Geometry check sheet. Reference: the model listing, model coordinates, mm. Face numbers are marked on the shaded views. Round coordinates to 2 decimals unless told otherwise and drop trailing zeros. Loops run counter-clockwise (first coordinate to the right, second up) from the corner with the lowest first, then second, coordinate; pieces in that order, holes last. Notation, with made-up numbers: (-13.5, -38.5) -> (18.5, -38.5) arc R21 ccw to (18.5, -21.5) -> close; hole circle Ø11 at (78.5, 38.5). An arc over 180 degrees is marked (long way). Use a Markdown table: item, result. Add a question column.
Q1. Sectioned sample at B-B, the plane x = -0.5. Give the number of separate pieces and of enclosed holes in the cut face, then the cut area to 3 significant figures.
Q2. Material ranges on L1, parallel to Z at x = -0.5, y = 1.9; L2, parallel to X at y = 1.95, z = 17.5; L3, parallel to Z at x = -0.5, y = 4.5, recorded low to high.
Q3. Sectioned sample at D-D, the plane z = 29. Enter the section's corners in (x, y), then the cut area to 3 significant figures.
Q4. Sectioned sample at C-C, the plane y = 6.25. Enter the section's corners in (x, z), then the cut area to 3 significant figures.
Q5. Gauge pin test, flat ends, axial feed: P1, Ø1, axis at y = 5, z = -16, coming from the +X side; P2, Ø5, axis at x = -1, z = -17.5, coming from the +Y side. Record the tip position at first contact, or that the pin passes through.
Q6. Release check for a two-part mould opening along Z. For the marked faces 1, 2, 3 and 4 record: released by +Z, released by -Z, zero draft, split by the parting line, or undercut.
Q7. Sectioned sample at A-A, the plane z = -6.5. Enter the section's corners in (x, y).
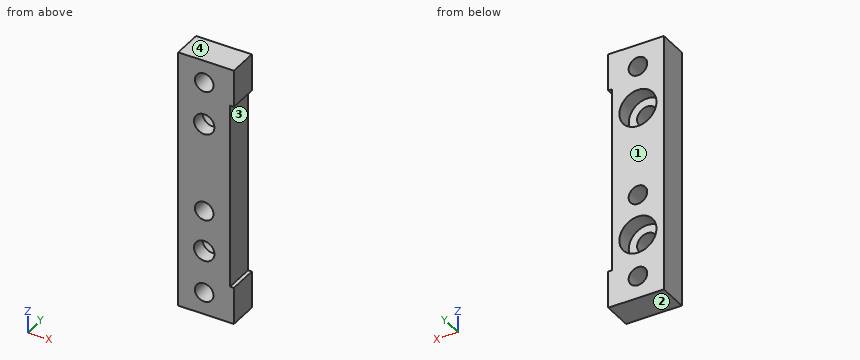
```python
from build123d import *

# Parameters (mm, degrees)
SKETCH1_W           = 15
SKETCH1_H           = 70
BOSS_EXTRUDE1_DEPTH = 8
SKETCH2_W           = 1
SKETCH2_H           = 50
CUT_EXTRUDE1_DEPTH  = 8
SKETCH3_R           = 2.5
CUT_EXTRUDE2_DEPTH  = 8
SKETCH4_R           = 2.75
CUT_EXTRUDE3_DEPTH  = 8
SKETCH5_R           = 5
CUT_EXTRUDE4_DEPTH  = 4.2
SKETCH6_R           = 2.5
CUT_EXTRUDE5_DEPTH  = 72.2


with BuildPart() as part:
    # Sketch1 → Boss-Extrude1 (new body)
    with BuildSketch(Plane(origin=(0, 0, 0), x_dir=(1, 0, 0), z_dir=(0, 1, 0))):
        Rectangle(SKETCH1_W, SKETCH1_H)
    extrude(amount=BOSS_EXTRUDE1_DEPTH)

    # Sketch2 → Cut-Extrude1 (cut)
    with BuildSketch(Plane(origin=(0, 8, 0), x_dir=(1, 0, 0), z_dir=(0, 1, 0))):
        with Locations((7, 0)):
            Rectangle(SKETCH2_W, SKETCH2_H)
    extrude(amount=-CUT_EXTRUDE1_DEPTH, mode=Mode.SUBTRACT)

    # Sketch3 → Cut-Extrude2 (cut)
    with BuildSketch(Plane(origin=(0, 8, 0), x_dir=(1, 0, 0), z_dir=(0, 1, 0))):
        with Locations((-0.5, -29)):
            Circle(SKETCH3_R)
        with Locations((-0.5, 29)):
            Circle(SKETCH3_R)
    extrude(amount=-CUT_EXTRUDE2_DEPTH, mode=Mode.SUBTRACT)

    # Sketch4 → Cut-Extrude3 (cut)
    with BuildSketch(Plane(origin=(0, 8, 0), x_dir=(1, 0, 0), z_dir=(0, 1, 0))):
        with Locations((-0.5, -17.5)):
            Circle(SKETCH4_R)
        with Locations((-0.5, 17.5)):
            Circle(SKETCH4_R)
    extrude(amount=-CUT_EXTRUDE3_DEPTH, mode=Mode.SUBTRACT)

    # Sketch5 → Cut-Extrude4 (cut)
    with BuildSketch(Plane(origin=(0, 8, 0), x_dir=(1, 0, 0), z_dir=(0, 1, 0))):
        with Locations((-0.5, 17.5)):
            Circle(SKETCH5_R)
        with Locations((-0.5, -17.5)):
            Circle(SKETCH5_R)
    extrude(amount=-CUT_EXTRUDE4_DEPTH, mode=Mode.SUBTRACT)

    # Sketch6 → Cut-Extrude5 (cut)
    with BuildSketch(Plane(origin=(0, 8, 0), x_dir=(1, 0, 0), z_dir=(0, 1, 0))):
        with Locations((-0.5, 6.5)):
            Circle(SKETCH6_R)
    extrude(amount=-CUT_EXTRUDE5_DEPTH, mode=Mode.SUBTRACT)


solid = part.part
```
Values:
| question | item | result |
|---|---|---|
| 1 | separate pieces | 6 |
| 1 | enclosed holes | 0 |
| 1 | area | 314 mm^2 |
| 2 | L1 | -35 to -31.5, -26.5 to -20.25, -14.75 to -9, -4 to 14.75, 20.25 to 26.5, 31.5 to 35 |
| 2 | L2 | -7.5 to -3.25, 2.25 to 6.5 |
| 2 | L3 | -35 to -31.5, -26.5 to -22.5, -12.5 to -9, -4 to 12.5, 22.5 to 26.5, 31.5 to 35 |
| 3 | outline | (-7.5, 0) -> (-3, 0) -> (-3, 8) -> (-7.5, 8) -> close; (2, 0) -> (7.5, 0) -> (7.5, 8) -> (2, 8) -> close |
| 3 | area | 80.0 mm^2 |
| 4 | outline | (-7.5, -35) -> (7.5, -35) -> (7.5, -25) -> (6.5, -25) -> (6.5, 25) -> (7.5, 25) -> (7.5, 35) -> (-7.5, 35) -> close; hole circle Ø10 at (-0.5, -17.5); hole circle Ø10 at (-0.5, 17.5); hole circle Ø5 at (-0.5, -29); hole circle Ø5 at (-0.5, -6.5); hole circle Ø5 at (-0.5, 29) |
| 4 | area | 784 mm^2 |
| 5 | P1 | x = 6.5 |
| 5 | P2 | y = 3.8 |
| 6 | face 1 | zero draft |
| 6 | face 2 | released by -Z |
| 6 | face 3 | undercut |
| 6 | face 4 | released by +Z |
| 7 | outline | (-7.5, 0) -> (-3, 0) -> (-3, 8) -> (-7.5, 8) -> close; (2, 0) -> (6.5, 0) -> (6.5, 8) -> (2, 8) -> close |
